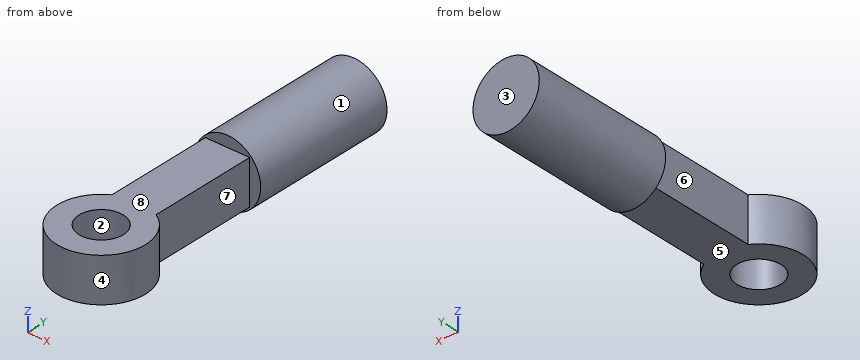
from build123d import *

# Parameters (mm, degrees)
CROQUIS1_R              = 1.5
SALIENTE_EXTRUIR1_DEPTH = 3
CROQUIS2_R              = 2.25
SALIENTE_EXTRUIR2_DEPTH = 10


with BuildPart() as part:
    # Croquis1 → Saliente-Extruir1 (new body)
    with BuildSketch(Plane.XY):
        with BuildLine():
            Line((1.5, 10), (-1.5, 10))
            Line((-1.5, 10), (-1.5, 2.598076211))
            ThreePointArc((-1.5, 2.598076211), (0, -3), (1.5, 2.598076211))
            Line((1.5, 2.598076211), (1.5, 10))
        make_face()
        Circle(CROQUIS1_R, mode=Mode.SUBTRACT)
    extrude(amount=SALIENTE_EXTRUIR1_DEPTH)

    # Croquis2 → Saliente-Extruir2 (add)
    with BuildSketch(Plane(origin=(0, 10, 0), x_dir=(1, 0, 0), z_dir=(0, 1, 0))):
        with Locations(Location((0, -1.5, 0), (0, 0, 270))):
            Circle(CROQUIS2_R)
    extrude(amount=SALIENTE_EXTRUIR2_DEPTH)


solid = part.part
Source: CAD feature listing. Evaluate the final solid. Frame: model axes, mm. Face numbers are marked on the shaded views. A direction names the side the tool comes from. Give positions to 0.01 mm unless a question says otherwise; leave off trailing zeros. Order: outer loops, then holes, each group sorted by start corner. A loop starts at its lowest first (then second) coordinate and runs counter-clockwise, first axis right, second up. Notation, with made-up numbers: (3.25, 44.5) -> (51.25, 44.5) arc R21 ccw to (51.25, 73.5) -> close; hole circle Ø10 at (-17, 35.25). An arc over 180 degrees is marked (long way). Write item = value, one per line.
Item 1: Section query D-D (y = 7.5). Output: boundary loops of the cut face in (x, z), then the cut area to 3 significant figures.
Check result:
outline = (-1.5, 0) -> (1.5, 0) -> (1.5, 3) -> (-1.5, 3) -> close
area = 9.00 mm²
Item 2: Section query C-C (y = 0). Output: boundary loops of the cut face in (x, z).
Check result:
outline = (-3, 0) -> (-1.5, 0) -> (-1.5, 3) -> (-3, 3) -> close; (1.5, 0) -> (3, 0) -> (3, 3) -> (1.5, 3) -> close
Item 3: Set-up query: the marked faces 4, 5, 6, 7 and 8. Return all of +Z, -Z, +X, -X, +Y, -Y with unobstructed straight access to the full face (end or side cutting, diameter ignored); none if empty.
Check result:
face_4 = +Z, -Z
face_5 = -Z, +X, -X, -Y
face_6 = +Z, -Z, -X
face_7 = +Z, -Z, +X
face_8 = +Z, +X, -X, -Y
Item 4: Section query A-A (x = 0). Output: boundary loops of the cut face in (y, z), then the cut area to 3 significant figures.
Check result:
outline = (-3, 0) -> (-1.5, 0) -> (-1.5, 3) -> (-3, 3) -> close; (1.5, 0) -> (10, 0) -> (10, -0.75) -> (20, -0.75) -> (20, 3.75) -> (10, 3.75) -> (10, 3) -> (1.5, 3) -> close
area = 75.0 mm²
Item 5: Section query B-B (z = 1.5). Output: boundary loops of the cut face in (x, y), then the cut area to 3 significant figures.
Check result:
outline = (-2.25, 10) -> (-1.5, 10) -> (-1.5, 2.6) arc R3 ccw (long way) to (1.5, 2.6) -> (1.5, 10) -> (2.25, 10) -> (2.25, 20) -> (-2.25, 20) -> close; hole circle Ø3 at (0, 0)
area = 87.6 mm²
Item 6: Ray query, probe 1 along Y at (x, z) = (0, 1.1); probe 2 along Z at (x, y) = (0.7, -1.5); probe 3 along Y at (x, z) = (1.05, -0.45). Return the intervals inside material, ascending.
Check result:
probe_1 = -3 to -1.5, 1.5 to 20
probe_2 = 0 to 3
probe_3 = 10 to 20
Item 7: Mould query, pull axis Y, two halves, no side actions, for the marked faces 1, 2 and 3. Classes: +Y half, -Y half, draft (parallel to the pull), parting line (faces both ways), or undercut.
Check result:
face_1 = draft
face_2 = undercut
face_3 = +Y half
Item 8: Contact query for flat-ended pins moving along their axis: pin 1 (1.5 mm diameter, centred on y = 7, z = 1.5, fed in from -X); pin 2 (1.8 mm diameter, centred on x = -1, y = 1.5, fed in from +Z); pin 3 (2.5 mm diameter, centred on y = 6.5, z = 1, fed in from +X). Output: stop coordinate, or through.
Check result:
pin_1 = -1.5
pin_2 = 3
pin_3 = 1.5
